Geometry: see drawing. Coordinates: mm, zero at the bounding-box minimum. Give positions to 0.01 mm unless a question says otherwise; leave off trailing zeros. Write each loop counter-clockwise with the first axis right and the second up, starting at its lowest first coordinate (ties: lowest second). Pieces come first, ordered by that corner, then holes. Notation, with made-up numbers: (38, -34) - (46, -34) arc R31 ccw to (46, -5) - close; hole circle Ø6 at (-31, -29.5). An arc over 180 degrees is marked (long way). Answer as CSV lines item,"result". Start each with the question number.
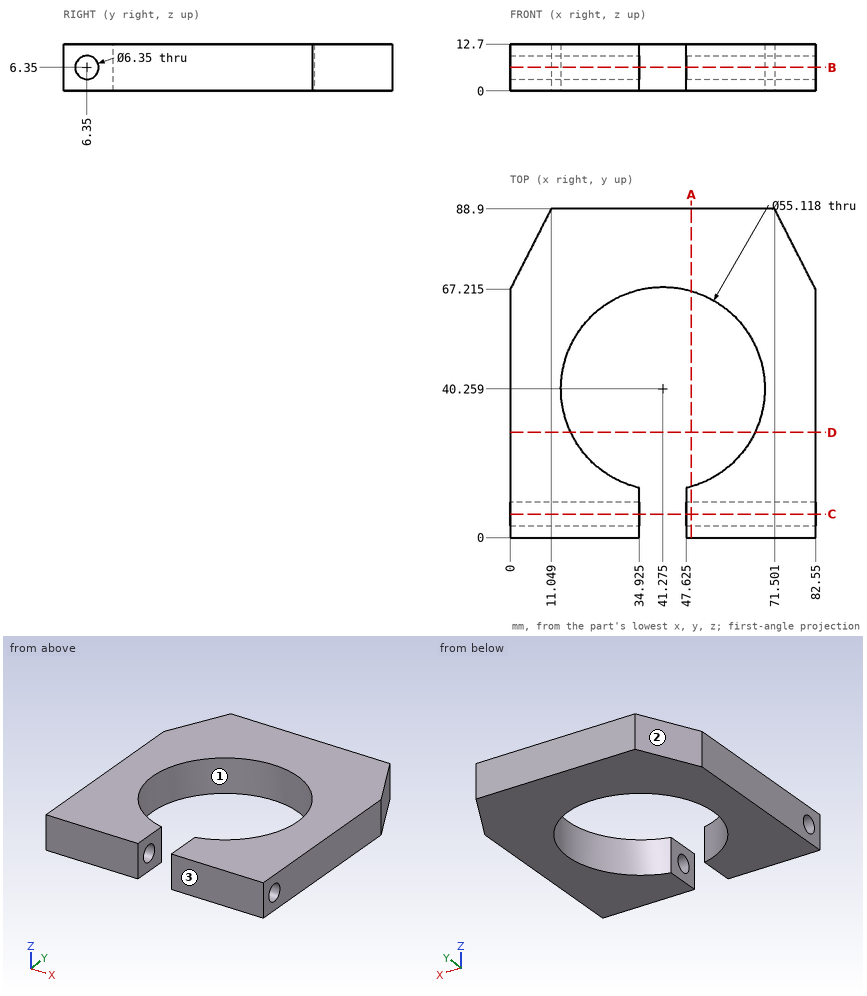
1) Cut plane B-B on z = 6.35. State how many separate pieces and enclosed holes the cut face has, and give its area (4 significant figures).
2) Contact query for a flat-ended pin moving along its axis: P1, Ø6, axis at x = 54, z = 10, coming from the -Y side. Output: stop coordinate, or through.
3) Cut plane C-C on y = 6.35. Output: boundary loops of the cut face in (x, z) (3 decimals).
4) Cut plane D-D on y = 28.5. Output: boundary loops of the cut face in (x, z), and give its area (3 significant figures).
5) Cut plane A-A on x = 49. Output: boundary loops of the cut face in (y, z) (3 decimals), and give its area (3 significant figures).
6) Pull-direction query (X, two-part tool) for the marked faces 1, 2 and 3; classes: +X half, -X half, draft (parallel to the pull), parting line (faces both ways), or undercut.
7) Material intervals for line 1 (Z direction, x = 23, y = 6.35) (3 decimals); line 2 (Y direction, x = 28, z = 6); line 3 (Y direction, x = 54.5, z = 7.25) (1 decimal), sorted ascending. Write a range as from..to.
Numbers:
1,separate pieces,"3"
1,enclosed holes,"0"
1,area,"4,105 mm²"
2,P1,"stops at y = 0"
3,outline,"(0, 0) - (34.925, 0) - (34.925, 3.175) - (0, 3.175) - close; (0, 9.525) - (34.925, 9.525) - (34.925, 12.7) - (0, 12.7) - close; (47.625, 0) - (82.55, 0) - (82.55, 3.175) - (47.625, 3.175) - close; (47.625, 9.525) - (82.55, 9.525) - (82.55, 12.7) - (47.625, 12.7) - close"
4,outline,"(0, 0) - (16.35, 0) - (16.35, 12.7) - (0, 12.7) - close; (66.2, 0) - (82.55, 0) - (82.55, 12.7) - (66.2, 12.7) - close"
4,area,"415 mm²"
5,outline,"(0, 0) - (13.805, 0) - (13.805, 12.7) - (0, 12.7) - close; (66.713, 0) - (88.9, 0) - (88.9, 12.7) - (66.713, 12.7) - close; hole circle Ø6.35 at (6.35, 6.35)"
5,area,"425 mm²"
6,face 1,"undercut"
6,face 2,"-X half"
6,face 3,"draft"
7,line 1,"z = 0..3.175, 9.525..12.7"
7,line 2,"y = 0..3.19, 9.51..16.11, 64.41..88.9"
7,line 3,"y = 0..3.3, 9.4..16.1, 64.4..88.9"
